Check sheet for the modelled part. Datum: model origin and axes. Units: mm. A direction names the side the tool comes from. Round coordinates to 2 decimals unless told otherwise and drop trailing zeros. Loops run counter-clockwise (first coordinate to the right, second up) from the corner with the lowest first, then second, coordinate; pieces in that order, holes last. Notation, with made-up numbers: (-20, -32.5) - (33, -32.5) arc R18 cw to (33, -27.5) - close; hole circle Ø7 at (40.25, 20.5). An arc over 180 degrees is marked (long way). Put each result on its own line as item: value. Start each with the question number.
Item 1: Gauge pin test, flat ends, axial feed: pin 1 Ø3.5 at (x, z) = (-564.58, -29.61) entering from +Y; pin 2 Ø1 at (x, z) = (326, 24.5) entering from +Y. Record the tip position at first contact, or that the pin passes through.
Item 2: Section check A-A, the plane y = 14. Record the cut outline in (x, z), and give its area (3 significant figures).
Item 3: Tool access check on faces 1 (the flat face through (-592.53, -1, 14)), 2 (the flat face through (48, 27, -40.108)). Record the directions out of +Z, -Z, +X, -X, +Y, -Y that give a thin tool (end or side, any length) a straight path to the whole face; none if there is none.
Item 4: Material ranges on line 1 along Z through (x, y) = (-202, 38.5); line 2 along Y through (x, z) = (-488, -9), recorded low to high.
Item 5: Section check C-C, the plane z = -5.5. Record the cut outline in (x, y).
Item 6: Section check B-B, the plane x = 250. Record the cut outline in (y, z).
from build123d import *

# Parameters (mm, degrees)
CROQUIS1_W                      = 1300
CROQUIS1_H                      = 220
BRIDA_BASE1_DEPTH               = 1.5
PLIEGUE_START                   = -592.530487805
PLIEGUE_CROQUIZADO1_DEPTH       = 1300
PLIEGUE_CROQUIZADO1_2_OUTLINE_W = 55.321902755
PLIEGUE_CROQUIZADO1_2_OUTLINE_H = 1.5
PLIEGUE_CROQUIZADO1_2_DEPTH     = 1300
CROQUIS8_R                      = 3
CORTAR_EXTRUIR1_DEPTH           = 10


# Read off the part's stored shape, not the designer's step: Pliegue croquizado1
# Sheet-metal steps are written as plain solids
with BuildPart() as part:
    # Croquis1 → Brida base1 (new body)
    with BuildSketch(Plane(origin=(0, 0, 0), x_dir=(1, 0, 0), z_dir=(0, 1, 0))):
        with Locations((57.469512195, -13.391768293)):
            Rectangle(CROQUIS1_W, CROQUIS1_H)
    extrude(amount=-BRIDA_BASE1_DEPTH)

    # Pliegue croquizado1 outline → Pliegue croquizado1 (cut)
    with BuildSketch(Plane.YZ.offset(PLIEGUE_START)):
        with BuildLine():
            Line((0, -96.608231707), (0, -41.608231707))
            ThreePointArc((0, -41.608231707), (-1.060660172, -41.168891879), (-1.5, -40.108231707))
            Line((-1.5, -40.108231707), (-1.5, -96.608231707))
            Line((-1.5, -96.608231707), (0, -96.608231707))
        make_face()
        with BuildLine():
            Line((-1.5, 123.391768293), (-1.5, 66.891768293))
            ThreePointArc((-1.5, 66.891768293), (-1.060660171, 67.952428465), (0, 68.391768293))
            Line((0, 68.391768293), (0, 123.391768293))
            Line((0, 123.391768293), (-1.5, 123.391768293))
        make_face()
    extrude(amount=PLIEGUE_CROQUIZADO1_DEPTH, mode=Mode.SUBTRACT)

    # Pliegue croquizado1 2 outline → Pliegue croquizado1 2 (add)
    with BuildSketch(Plane.YZ.offset(PLIEGUE_START)):
        with Locations((27.660951378, -40.858231707)):
            Rectangle(PLIEGUE_CROQUIZADO1_2_OUTLINE_W, PLIEGUE_CROQUIZADO1_2_OUTLINE_H)
        with Locations((27.660951378, 67.641768293)):
            Rectangle(PLIEGUE_CROQUIZADO1_2_OUTLINE_W, PLIEGUE_CROQUIZADO1_2_OUTLINE_H)
    extrude(amount=PLIEGUE_CROQUIZADO1_2_DEPTH)

    # Croquis8 → Cortar-Extruir1 (cut)
    with BuildSketch(Plane(origin=(0, 0, 0), x_dir=(1, 0, 0), z_dir=(0, 1, 0))):
        with Locations(Location((-564.580402517, -56.391768293, 0), (0, 0, 270))):
            Circle(CROQUIS8_R)
        with Locations(Location((-540.580402517, -56.391768293, 0), (0, 0, 270))):
            Circle(CROQUIS8_R)
        with Locations(Location((-540.580402517, 29.608231707, 0), (0, 0, 270))):
            Circle(CROQUIS8_R)
        with Locations(Location((-564.580402517, 29.608231707, 0), (0, 0, 270))):
            Circle(CROQUIS8_R)
    extrude(amount=-CORTAR_EXTRUIR1_DEPTH, mode=Mode.SUBTRACT)


solid = part.part
Check result:
1. pin 1: through
1. pin 2: y = 0
2. outline: (-592.53, -41.61) - (707.47, -41.61) - (707.47, -40.11) - (-592.53, -40.11) - close; (-592.53, 66.89) - (707.47, 66.89) - (707.47, 68.39) - (-592.53, 68.39) - close
2. area: 3,900 mm²
3. face 1: +Z, -Z, -X, +Y, -Y
3. face 2: +X, -X, +Y
4. line 1: -41.61 to -40.11, 66.89 to 68.39
4. line 2: -1.5 to 0
5. outline: (-592.53, -1.5) - (707.47, -1.5) - (707.47, 0) - (-592.53, 0) - close
6. outline: (-1.5, -40.11) arc R1.5 ccw to (0, -41.61) - (55.32, -41.61) - (55.32, -40.11) - (0, -40.11) - (0, 66.89) - (55.32, 66.89) - (55.32, 68.39) - (0, 68.39) arc R1.5 ccw to (-1.5, 66.89) - close
